Read the model definition and answer for the solid it produces. Units are mm, in the model's axes. A direction names the side the tool comes from. Coordinates: 2 decimals unless noted, no trailing zeros. Write each loop counter-clockwise with the first axis right and the second up, starting at its lowest first coordinate (ties: lowest second). Pieces come first, ordered by that corner, then holes.
1) The part is cut by section D-D (y = 62). Determine the outline of the cut face in (x, z).
2) Determine the mould class of faces 1 (the face through (0, 27, 2)), 2 (the face through (-7.5, 18, 1)), 3 (the face through (6.9, 5.57, 1.52)) for opening direction Y: +Y half, -Y half, draft (parallel to the pull), parting line (faces both ways), or undercut.
3) Which of the six approach directions +Z, -Z, +X, -X, +Y, -Y give full straight-line access (tool end or side, diameter ignored) to faces 4 (the face through (0.22, 44.19, 1.48)), 5 (the face through (0, 5, 1))?
4) Each of these flat-tipped pins is pushed along its axis until it touches: pin 1 Ø0.9 at (y, z) = (16, 2) entering from -X; pin 2 Ø1 at (x, z) = (-1, 1) entering from +Y. Where does it stop, or does it pass through?
5) Find the intervals of material crossed by line 1 (Y direction, x = 0, z = 2.6); line 2 (X direction, y = 64, z = 2.8); line 3 (Y direction, x = -2.5, z = 1.65), in increasing order.
6) The part is cut by section A-A (y = 76.5). Determine the outline of the cut face in (x, z).
7) The part is cut by section C-C (z = 0.6). Give the number of separate pieces and of enclosed holes in the cut face, then the cut area to 3 significant figures.
8) The part is cut by section B-B (x = 0). Determine the outline of the cut face in (y, z), then the cut area to 3 significant figures.
Autodesk Inventor part; units mm, degrees
ref_plane "YZ Plane" through (0, 0, 0) normal (1, 0, 0) x (0, 1, 0)
ref_plane "XZ Plane" through (0, 0, 0) normal (0, 1, 0) x (-1, 0, 0)
ref_plane "XY Plane" through (0, 0, 0) normal (0, 0, 1) x (1, 0, 0)
sketch "Эскиз1" plane through (0, 0, 0) normal (0, 0, 1) x (1, 0, 0)
  line L0 (17.5, 5) -> (-17.5, 5) construction
  line L1 (-17.5, 5) -> (-17.5, -5) construction
  line L2 (-17.5, -5) -> (17.5, -5) construction
  line L3 (17.5, -5) -> (17.5, 5) construction
  line L4 (17.5, 5) -> (-17.5, -5) construction
  line L5 (-17.5, 5) -> (17.5, -5) construction
  line L6 (12.8471, 5) -> (-11.1661, 5) construction
  circle A0 centre (0, 64.187) radius 35
  circle A1 centre (0, 64.187) radius 20
  line L7 (0, 64.187) -> (0, 0) construction
  circle A2 centre (0, 88.737) radius 4.55
  line L8 (-7.5, 5) -> (-7.5, 30)
  line L9 (7.5, 30) -> (7.5, 5)
  line L10 (-2, 49.2906) -> (2, 49.2906) construction
  line L11 (-7.5, 5) -> (7.5, 5)
  line L12 (-2, 85.687) -> (2, 85.687)
  line L13 (2, 85.687) -> (2, 82.687)
  line L14 (2, 82.687) -> (-2, 82.687)
  line L15 (-2, 82.687) -> (-2, 85.687)
  line L16 (-2, 85.687) -> (2, 82.687) construction
  line L17 (2, 85.687) -> (-2, 82.687) construction
  line L18 (-17.6195, 51.7049) -> (-19.6195, 55.169)
  circle A3 centre (-21.2609, 51.912) radius 4.55
  line L19 (-17.0215, 56.669) -> (-15.0215, 53.2049)
  line L20 (-19.6195, 55.169) -> (-17.0215, 56.669)
  line L21 (-15.0215, 53.2049) -> (-17.6195, 51.7049)
  line L22 (19.6195, 55.169) -> (17.6195, 51.7049)
  circle A4 centre (21.2609, 51.912) radius 4.55
  line L23 (15.0215, 53.2049) -> (17.0215, 56.669)
  line L24 (17.6195, 51.7049) -> (15.0215, 53.2049)
  line L25 (17.0215, 56.669) -> (19.6195, 55.169)
  point P0 (0, 89.2906)
  point P1 (0, 84.187)
  point P2 (-17.3205, 54.187)
  point P3 (17.3205, 54.187)
  point P4 (18.2337, 55.9692)
  point P5 (18.7216, 55.6875)
  point P6 (16.7216, 52.2234)
  point P7 (16.2337, 52.5051)
  point P8 (-16.2337, 52.5051)
  point P9 (-16.7216, 52.2234)
  point P10 (-18.7216, 55.6875)
  point P11 (-18.2337, 55.9692)
  point P12 (-2, 84.0867)
  point P13 (-2, 84.6501)
  point P14 (2, 84.6501)
  point P15 (2, 84.0867)
  dimension "d3" = 40
  dimension "d4" = 9.1
  dimension "d0" = 70
  dimension "d9" = 35
  dimension "d10" = 25
  dimension "d11" = 10
  dimension "d12" = 15
  dimension "d14" = 7.5
  dimension "d30" = 4
  dimension "d31" = 3
  dimension "d34" = 360
extrude "Выдавливание1" add sketch "Эскиз1" along normal blind 3
fillet "Сопряжение1" radius 2 14 edges at (-7.5, 30, 1.5) (7.5, 30, 1.5) (-18.2337, 55.9692, 1.5) (-18.7216, 55.6875, 1.5) (-16.2337, 52.5051, 1.5) (-16.7216, 52.2234, 1.5) (-2, 84.0867, 1.5) (-2, 84.6501, 1.5) (2, 84.0867, 1.5) (2, 84.6501, 1.5) (18.7216, 55.6875, 1.5) (18.2337, 55.9692, 1.5) (16.7216, 52.2234, 1.5) (16.2337, 52.5051, 1.5)
sketch "Эскиз2" plane through (0, 0, 3) normal (0, 0, 1) x (1, 0, 0)
  circle A0 centre (0, 25) radius 2 construction
  circle A1 centre (0, 10) radius 2 construction
  line L0 (0, 0) -> (0, 43.9437)
  line L1 (0, 10) -> (0, 5)
  line L2 (-7.5, 5) -> (7.5, 5)
  arc A2 (19.3109, 58.9824) -> (5.1482, 83.513) centre (0, 64.187) ccw
  arc A3 (-3.1613, 25.1277) -> (3.1613, 25.1277) centre (0, 64.187) ccw construction
  arc A4 (-3.3227, 23.1342) -> (3.3227, 23.1342) centre (0, 64.187) ccw
  arc A5 (-3, 27.1212) -> (3, 27.1212) centre (0, 64.187) ccw
  arc A6 (-3, 27.1212) -> (-3.3227, 23.1342) centre (-3.1613, 25.1277) ccw
  arc A7 (3.3227, 23.1342) -> (3, 27.1212) centre (3.1613, 25.1277) ccw
  arc A8 (-3.115, 10.0896) -> (3.115, 10.0896) centre (0, 64.187) ccw construction
  arc A9 (-3.2299, 8.0929) -> (3.2299, 8.0929) centre (0, 64.187) ccw
  arc A10 (-3, 12.0863) -> (3, 12.0863) centre (0, 64.187) ccw
  arc A11 (-3, 12.0863) -> (-3.2299, 8.0929) centre (-3.115, 10.0896) ccw
  arc A12 (3.2299, 8.0929) -> (3, 12.0863) centre (3.115, 10.0896) ccw
  dimension "d24" = 15
  dimension "d25" = 5
  dimension "d26" = 4
  dimension "d27" = 4
  dimension "d39" = 4
  dimension "d40" = 6
  dimension "d41" = 4
  dimension "d42" = 6
extrude "Выдавливание2" cut sketch "Эскиз2" against normal blind 4
fillet "Сопряжение2" radius 2 2 edges at (7.5, 5, 1.5) (-7.5, 5, 1.5)
properties part number "Деталь2_мозговорот"
Reported:
1. outline: (-34.93, 0) - (-19.88, 0) - (-19.88, 3) - (-34.93, 3) - close; (19.88, 0) - (34.93, 0) - (34.93, 3) - (19.88, 3) - close
2. face 1: undercut
2. face 2: draft
2. face 3: -Y half
3. face 4: +Z, -Z
3. face 5: +Z, -Z, +X, -X, -Y
4. pin 1: stops at x = -7.5
4. pin 2: stops at y = 99.18
5. line 1: y = 5 to 8, 12 to 23, 27 to 44.19, 93.29 to 99.19
5. line 2: x = -35 to -20, 20 to 35
5. line 3: y = 5 to 8.06, 12.06 to 23.08, 27.08 to 44.34, 92.54 to 99.1
6. outline: (-32.76, 0) - (-15.76, 0) - (-15.76, 3) - (-32.76, 3) - close; (15.76, 0) - (32.76, 0) - (32.76, 3) - (15.76, 3) - close
7. separate pieces: 1
7. enclosed holes: 3
7. area: 2,670 mm2
8. outline: (5, 0) - (8, 0) - (8, 3) - (5, 3) - close; (12, 0) - (23, 0) - (23, 3) - (12, 3) - close; (27, 0) - (44.19, 0) - (44.19, 3) - (27, 3) - close; (93.29, 0) - (99.19, 0) - (99.19, 3) - (93.29, 3) - close
8. area: 111 mm2
